Autodesk Inventor part; units mm, degrees
ref_plane "YZ Plane" through (0, 0, 0) normal (1, 0, 0) x (0, 1, 0)
ref_plane "XZ Plane" through (0, 0, 0) normal (0, 1, 0) x (-1, 0, 0)
ref_plane "XY Plane" through (0, 0, 0) normal (0, 0, 1) x (1, 0, 0)
sketch "Sketch1" plane through (0, 0, 0) normal (0, 1, 0) x (-1, 0, 0)
  line L0 (70, -85) -> (5, -85)
  line L1 (5, -85) -> (5, -15)
  line L2 (5, -15) -> (70, -15)
  line L3 (70, -15) -> (70, -85)
  line L4 (73, -15) -> (73, -85)
  line L5 (73, -85) -> (73, -88)
  line L6 (73, -88) -> (5, -88)
  line L7 (5, -88) -> (2, -88)
  line L8 (2, -88) -> (2, -15)
  line L9 (2, -15) -> (2, -12)
  line L10 (2, -12) -> (73, -12)
  line L11 (73, -12) -> (73, -15)
  line L12 (70, -85) -> (5, -85)
  line L13 (5, -85) -> (5, -15)
  line L14 (5, -15) -> (70, -15)
  line L15 (70, -15) -> (70, -85)
  line L16 (73, -88) -> (2, -88)
  line L17 (2, -88) -> (2, -12)
  line L18 (2, -12) -> (73, -12)
  line L19 (73, -12) -> (73, -88)
  point P0 (0, 0)
  dimension "d25" = 70
extrude "Extrusion1" add sketch "Sketch1" against normal blind 35
sketch "Sketch2" plane through (0, 0, 0) normal (0, 1, 0) x (1, 0, 0)
  line L0 (-2, 12) -> (-2, 88)
  line L1 (-2, 12) -> (-73, 12)
  line L2 (-73, 12) -> (-73, 88)
  line L3 (-73, 88) -> (-2, 88)
  line L4 (-2, 88) -> (-2, 12)
  point P0 (0, 0)
extrude "Extrusion2" add sketch "Sketch2" along normal blind 3
sketch "Sketch3" plane through (0, -35, 0) normal (0, -1, 0) x (1, 0, 0)
  line L0 (-73, -12) -> (-2, -12)
  circle A0 centre (-37.5, -12) radius 3
  line L1 (-73, -88) -> (-2, -88)
  circle A1 centre (-37.5, -88) radius 3
  line L2 (-73, -12) -> (-73, -88)
  circle A2 centre (-73, -50) radius 3
  line L3 (-2, -88) -> (-2, -12)
  circle A3 centre (-2, -50) radius 3
  point P0 (0, 0)
  point P1 (-34.5, -88)
  point P2 (-40.5, -88)
  point P3 (-73, -53)
  point P4 (-73, -47)
  dimension "d34" = 6
  dimension "d35" = 6
  dimension "d36" = 6
  dimension "d37" = 6
extrude "Extrusion3" add sketch "Sketch3" against normal blind 15 contours A0 L0 | L0 A0 | A3 L3 | L3 A3 | L2 A2 | A1 L1 picked at (-73.9927, -50.1205) picked at (-37.3795, -88.9927)
sketch "Sketch4" plane through (0, -35, 0) normal (0, -1, 0) x (1, 0, 0)
  line L0 (-73, -88) -> (-73, -12)
  circle A0 centre (-73, -50) radius 1.5
  arc A1 (-34.5, -12) -> (-40.5, -12) centre (-37.5, -12) ccw
  circle A2 centre (-37.5, -12) radius 1.5
  circle A3 centre (-37.5, -87.9085) radius 1.5
  line L1 (-2, -12) -> (-2, -88)
  circle A4 centre (-2, -50) radius 1.5
  point P0 (0, 0)
  dimension "d40" = 3
  dimension "d41" = 3
  dimension "d42" = 3
  dimension "d43" = 3
extrude "Extrusion4" cut sketch "Sketch4" against normal blind 7
properties part number "cajapic"
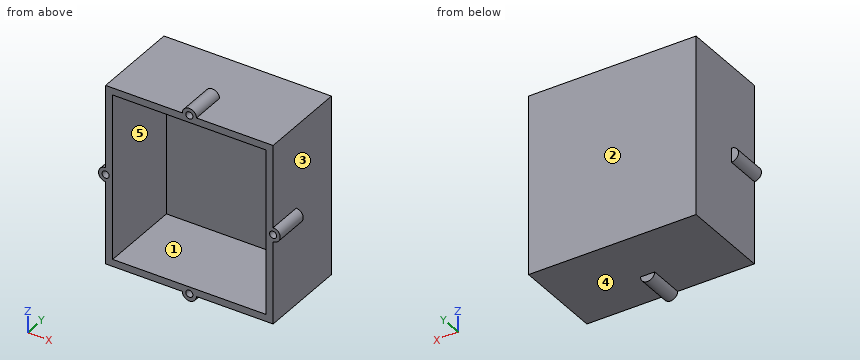
CAD build for the part. Positions are in the model's coordinates, mm. Face numbers are marked on the shaded views. A direction names the side the tool comes from. Coordinates: 2 decimals unless noted, no trailing zeros. Loops run counter-clockwise (first coordinate to the right, second up) from the corner with the lowest first, then second, coordinate; pieces in that order, holes last. Notation, with made-up numbers: (-39, 75) -> (-6, 75) arc R21 ccw to (-6, 109) -> close; hole circle Ø1 at (87, 29.25). An arc over 180 degrees is marked (long way). One line per item, written item: value.
1. Drill centre lines: line 1 (Z direction, x = -37.5, y = -29.75); line 2 (X direction, y = -32.5, z = -50); line 3 (X direction, y = -3, z = -31.5). Where is each one in solid material? Low to high. Write a range as [from, to].
Answers:
line 1: z = [-91, -89.41], [-86.41, -85], [-15, -13.5], [-10.5, -9]
line 2: x = [-76, -74.5], [-71.5, -70], [-5, -3.5], [-0.5, 1]
line 3: x = [-73, -70], [-5, -2]
2. Flat gauge pins, fed straight in: P1, Ø6, axis at y = -6, z = -39, coming from the -X side; P2, Ø2.5, axis at x = -2, z = -50, coming from the -Y side; P3, Ø10.5, axis at y = -10, z = -46.5, coming from the +X side. Where does each tip first touch, or does it go through?
Answers:
P1: stops at x = -73
P2: stops at y = -28
P3: stops at x = -2
3. Slice it at C-C on x = -68. Write the cut outline in (y, z), and give its area (3 significant figures).
Answers:
outline: (-35, -88) -> (3, -88) -> (3, -12) -> (-35, -12) -> (-35, -15) -> (0, -15) -> (0, -85) -> (-35, -85) -> close
area: 438 mm^2
4. Slice it at B-B on z = -16.5. Write the cut outline in (x, y).
Answers:
outline: (-73, -35) -> (-70, -35) -> (-70, 0) -> (-5, 0) -> (-5, -35) -> (-2, -35) -> (-2, 3) -> (-73, 3) -> close
5. Which spindle directions (+Z, -Z, +X, -X, +Y, -Y) get a long thin tool onto all of the face, cutting with end or side? Do the marked faces 1 and 2. Say none if no direction does.
Answers:
face 1: -Y
face 2: +Z, -Z, +X, -X, +Y
6. Slice it at A-A on y = -22. Write the cut outline in (x, z), and give its area (3 significant figures).
Answers:
outline: (-73, -88) -> (-40.5, -88) arc R3 ccw to (-34.5, -88) -> (-2, -88) -> (-2, -53) arc R3 ccw to (-2, -47) -> (-2, -12) -> (-34.5, -12) arc R3 ccw to (-40.5, -12) -> (-73, -12) -> (-73, -47) arc R3 ccw to (-73, -53) -> close; hole (-70, -85) -> (-5, -85) -> (-5, -15) -> (-70, -15) -> close
area: 903 mm^2
7. Slice it at D-D on y = -4.5. Write the cut outline in (x, z), and give its area (3 significant figures).
Answers:
outline: (-73, -88) -> (-2, -88) -> (-2, -12) -> (-73, -12) -> close; hole (-70, -85) -> (-5, -85) -> (-5, -15) -> (-70, -15) -> close
area: 846 mm^2
8. Pull direction X, two halves, no side cores. Call the marked faces 3, 4 and 5: pulls with the +X half, pulls with the -X half, needs draft (parallel to the pull), parting line crosses it, or undercut.
Answers:
face 3: pulls with the +X half
face 4: needs draft
face 5: undercut
